```python
from build123d import *

# Parameters (mm, degrees)
SKETCH6_R           = 51.2
BOSS_EXTRUDE4_DEPTH = 150
SKETCH7_R           = 24
CUT_EXTRUDE1_DEPTH  = 188.5


with BuildPart() as part:
    # Sketch6 → Boss-Extrude4 (new body)
    with BuildSketch(Plane.XY):
        Polygon((-250, -3.75), (-242.5, 3.75), (-103.75, 3.75), (-103.75, 168.75), (-88.75, 183.75), (88.75, 183.75), (103.75, 168.75), (103.75, 3.75), (242.5, 3.75), (250, -3.75), (250, -176.25), (242.5, -183.75), (-242.5, -183.75), (-250, -176.25), align=None)
        with Locations((0, 41.25)):
            Circle(SKETCH6_R, mode=Mode.SUBTRACT)
    extrude(amount=BOSS_EXTRUDE4_DEPTH)

    # Sketch7 → Cut-Extrude1 (cut, through all)
    with BuildSketch(Plane(origin=(0, 3.75, 0), x_dir=(1, 0, 0), z_dir=(0, 1, 0))):
        with Locations((-173.125, -75)):
            Circle(SKETCH7_R)
    cut_extrude1 = extrude(amount=-CUT_EXTRUDE1_DEPTH, mode=Mode.SUBTRACT)

    # Mirror1: Cut-Extrude1 across plane
    add(cut_extrude1.mirror(Plane(origin=(0, 0, 0), x_dir=(0, 0, 1), z_dir=(1, 0, 0))), mode=Mode.SUBTRACT)


solid = part.part
```
Input: part model. Units: mm. Frame: model coordinates. A direction names the side the tool comes from. Round coordinates to 2 decimals unless told otherwise and drop trailing zeros. Order: outer loops, then holes, each group sorted by start corner. A loop starts at its lowest first (then second) coordinate and runs counter-clockwise, first axis right, second up. Notation, with made-up numbers: (18, -34) - (75, -34) arc R22 ccw to (75, 4) - close; hole circle Ø2 at (-19, 15.25). An arc over 180 degrees is marked (long way). One line per question, with ' | ' between items. Start each with the question number.
1) Set-up query: faces 4 (the flat face through (250, -89, 74)), 5 (the flat face through (-103.75, 85, 74)), 6 (the flat face through (103.75, 87, 74)). Return all of +Z, -Z, +X, -X, +Y, -Y with unobstructed straight access to the full face (end or side cutting, diameter ignored); none if empty.
2) Ray query, probe 1 along X at (y, z) = (-144, 75) (3 decimals); probe 2 along Y at (x, z) = (0, 86); probe 3 along X at (y, z) = (-118.5, 66). Return the intervals inside material, ascending.
3) Cut plane D-D, the plane z = 18. Return the cut outline in (x, y), then the cut area to 3 significant figures.
4) Pull-direction query (Z, two-part tool) for faces 1 (the flat face through (-250, -91, 74)), 2 (the flat face through (3, -38, 150)), 3 (the cylindrical face through (-197.1, -88.7, 73.9)); classes: +Z half, -Z half, draft (parallel to the pull), parting line (faces both ways), or undercut.
5) Contact query for flat-ended pins moving along their axis: P1, Ø8, axis at x = -158, z = 15.5, coming from the +Y side; P2, Ø1.5, axis at y = 100.5, z = 59.5, coming from the +X side; P3, Ø1.5, axis at y = 119, z = 91.5, coming from the -X side. Output: stop coordinate, or through.
6) Cut plane C-C, the plane y = 41.25. Return the cut outline in (x, z).
7) Cut plane A-A, the plane z = 75. Return the cut outline in (x, y) (3 decimals), then the cut area to 3 significant figures.
8) Cut plane B-B, the plane x = 0. Return the cut outline in (y, z), then the cut area to 3 significant figures.
Worked out:
1) face 4: +Z, -Z, +X, +Y, -Y | face 5: +Z, -Z, -X, +Y | face 6: +Z, -Z, +X, +Y
2) probe 1: x = -250 to -197.125, -149.125 to 149.125, 197.125 to 250 | probe 2: y = -183.75 to -9.95, 92.45 to 183.75 | probe 3: x = -250 to -195.37, -150.88 to 150.88, 195.37 to 250
3) outline: (-250, -176.25) - (-242.5, -183.75) - (242.5, -183.75) - (250, -176.25) - (250, -3.75) - (242.5, 3.75) - (103.75, 3.75) - (103.75, 168.75) - (88.75, 183.75) - (-88.75, 183.75) - (-103.75, 168.75) - (-103.75, 3.75) - (-242.5, 3.75) - (-250, -3.75) - close; hole circle Ø102.4 at (0, 41.25) | area: 123,000 mm^2
4) face 1: draft | face 2: +Z half | face 3: undercut
5) P1: stops at y = 3.75 | P2: stops at x = 103.75 | P3: stops at x = -103.75
6) outline: (-103.75, 0) - (-51.2, 0) - (-51.2, 150) - (-103.75, 150) - close; (51.2, 0) - (103.75, 0) - (103.75, 150) - (51.2, 150) - close
7) outline: (-250, -176.25) - (-242.5, -183.75) - (-197.125, -183.75) - (-197.125, 3.75) - (-242.5, 3.75) - (-250, -3.75) - close; (-149.125, -183.75) - (149.125, -183.75) - (149.125, 3.75) - (103.75, 3.75) - (103.75, 168.75) - (88.75, 183.75) - (-88.75, 183.75) - (-103.75, 168.75) - (-103.75, 3.75) - (-149.125, 3.75) - close; (197.125, -183.75) - (242.5, -183.75) - (250, -176.25) - (250, -3.75) - (242.5, 3.75) - (197.125, 3.75) - close; hole circle Ø102.4 at (0, 41.25) | area: 105,000 mm^2
8) outline: (-183.75, 0) - (-9.95, 0) - (-9.95, 150) - (-183.75, 150) - close; (92.45, 0) - (183.75, 0) - (183.75, 150) - (92.45, 150) - close | area: 39,800 mm^2
